```python
from build123d import *

# Parameters (mm, degrees)
F0_W     = 64.9693608284
F0_H     = 45.7421503961
F1_DEPTH = 38.1
F3_DEPTH = 38.1
F4_R     = 6.35
F5_DEPTH = 25.4
F6_R     = 3.175
F7_DEPTH = 25.4


with BuildPart() as f1:
    # F0 (on Front) → F1 (new body)
    with BuildSketch(Plane.XZ):
        with Locations((32.4846804142, 22.8710751981)):
            Rectangle(F0_W, F0_H)
    extrude(amount=-F1_DEPTH)

    # F2 (on face) → F3 (cut)
    with BuildSketch(Plane.XY.offset(45.7421503961)):
        Polygon((38.1, 25.4), (0, 25.4), (0, 0), (64.9693608284, 0), (64.9693608284, 38.1), (38.1, 38.1), align=None)
    extrude(amount=-F3_DEPTH, mode=Mode.SUBTRACT)

    # F4 (on face) → F5 (cut)
    with BuildSketch(Plane.XZ.offset(-25.4)):
        with Locations((12.7, 33.0421503961)):
            Circle(F4_R)
        with BuildLine():
            ThreePointArc((12.6999999513, 45.7421503961), (21.6802561039, 42.0224065344), (25.4, 33.0421503961))
            Line((25.4, 33.0421503961), (25.4, 20.3421503961))
            ThreePointArc((25.4, 20.3421503961), (29.1197438789, 11.361894275), (38.1, 7.6421503961))
            Line((38.1, 7.6421503961), (38.1, 45.7421503961))
            Line((38.1, 45.7421503961), (12.6999999513, 45.7421503961))
        make_face()
        with BuildLine():
            ThreePointArc((0, 33.0421503961), (3.7197438617, 42.0224065), (12.6999999513, 45.7421503961))
            Line((12.6999999513, 45.7421503961), (0, 45.7421503961))
            Line((0, 45.7421503961), (0, 33.0421503961))
        make_face()
    extrude(amount=-F5_DEPTH, mode=Mode.SUBTRACT)

    # F6 (on face) → F7 (cut)
    with BuildSketch(Plane.XY.offset(7.6421503961)):
        with Locations((9.525, 9.525)):
            Circle(F6_R)
        with Locations((55.4443608284, 9.525)):
            Circle(F6_R)
        with Locations((55.4443608284, 28.575)):
            Circle(F6_R)
        with BuildLine():
            ThreePointArc((64.9693608284, 9.525), (62.1795529192, 2.7898079092), (55.4443608284, 0))
            Line((55.4443608284, 0), (64.9693608284, 0))
            Line((64.9693608284, 0), (64.9693608284, 9.525))
        make_face()
        with BuildLine():
            ThreePointArc((9.525, 0), (2.7898079092, 2.7898079092), (0, 9.525))
            Line((0, 9.525), (0, 0))
            Line((0, 0), (9.525, 0))
        make_face()
    extrude(amount=-F7_DEPTH, mode=Mode.SUBTRACT)


solid = f1.part
```
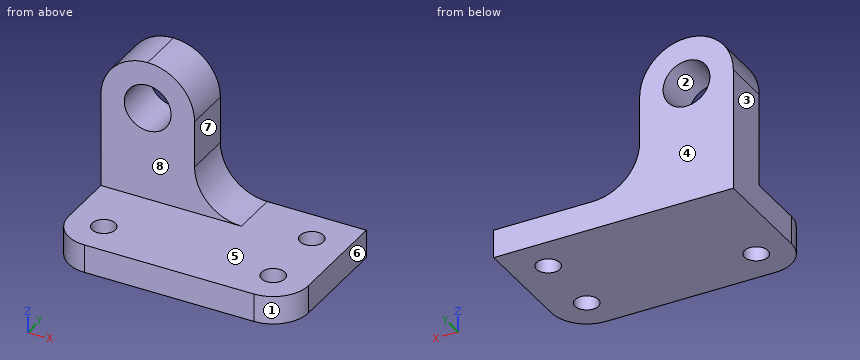
Geometry check sheet. Reference: the model listing, model coordinates, mm. Face numbers are marked on the shaded views. A direction names the side the tool comes from. Round coordinates to 2 decimals unless told otherwise and drop trailing zeros. Loops run counter-clockwise (first coordinate to the right, second up) from the corner with the lowest first, then second, coordinate; pieces in that order, holes last. Notation, with made-up numbers: (26.25, 34) -> (47.25, 34) arc R21 ccw to (47.25, 70) -> close; hole circle Ø9 at (-25.75, -35.75). An arc over 180 degrees is marked (long way). Use a Markdown table: item, result.
(1) Mould release check, pull along X, two halves, no side actions. Record for the marked faces 1, 2, 3 and 4: released by +X, released by -X, zero draft, split by the parting line, or undercut.
Calculated:
| item | result |
|---|---|
| face 1 | released by +X |
| face 2 | undercut |
| face 3 | released by -X |
| face 4 | zero draft |
(2) Sectioned sample at A-A (z = 34). Enter the section's corners in (x, y), then the cut area to 3 significant figures.
Calculated:
| item | result |
|---|---|
| outline | (0.04, 25.4) -> (6.42, 25.4) -> (6.42, 38.1) -> (0.04, 38.1) -> close; (18.98, 25.4) -> (25.36, 25.4) -> (25.36, 38.1) -> (18.98, 38.1) -> close |
| area | 162 mm² |
(3) Sectioned sample at D-D (x = 27.5). Enter the section's corners in (y, z).
Calculated:
| item | result |
|---|---|
| outline | (0, 0) -> (38.1, 0) -> (38.1, 13.35) -> (25.4, 13.35) -> (25.4, 7.64) -> (0, 7.64) -> close |
(4) Go/stop test with flat-tipped pins: P1, Ø8.5, axis at x = 9.525, y = 9.525, coming from the +Z side; P2, Ø6.5, axis at y = 31, z = 25.5, coming from the +X side; P3, Ø19, axis at x = 22, z = 31.5, coming from the -Y side. Record where each tip stops, or that it passes through.
Calculated:
| item | result |
|---|---|
| P1 | z = 7.64 |
| P2 | x = 25.4 |
| P3 | y = 25.4 |
(5) Sectioned sample at C-C (y = 21.5). Enter the section's corners in (x, z), then the cut area to 3 significant figures.
Calculated:
| item | result |
|---|---|
| outline | (0, 0) -> (64.97, 0) -> (64.97, 7.64) -> (0, 7.64) -> close |
| area | 497 mm² |
(6) Sectioned sample at B-B (z = 6.5). Enter the section's corners in (x, y) (3 decimals), then the cut area to 3 significant figures.
Calculated:
| item | result |
|---|---|
| outline | (0, 9.525) arc R9.525 ccw to (9.525, 0) -> (55.444, 0) arc R9.525 ccw to (64.969, 9.525) -> (64.969, 38.1) -> (0, 38.1) -> close; hole circle Ø6.35 at (9.525, 9.525); hole circle Ø6.35 at (55.444, 9.525); hole circle Ø6.35 at (55.444, 28.575) |
| area | 2,340 mm² |
(7) Scan lines: probe 1 along Z at (x, y) = (7.5, 24); probe 2 along X at (y, z) = (31, 21.5); probe 3 along X at (y, z) = (7.5, 6). Record each from-to range of solid material in increasing order.
Calculated:
| item | result |
|---|---|
| probe 1 | 0 to 7.64 |
| probe 2 | 0 to 25.4 |
| probe 3 | 0.22 to 7.08, 11.97 to 53, 57.89 to 64.75 |
(8) Set-up check for the marked faces 5, 6, 7 and 8: record each of +Z, -Z, +X, -X, +Y, -Y from which the full face is reachable in a straight line by a thin tool's end or side.
Calculated:
| item | result |
|---|---|
| face 5 | +Z, +X, -Y |
| face 6 | +Z, -Z, +X, +Y, -Y |
| face 7 | +Z, +X, +Y, -Y |
| face 8 | +Z, +X, -X, -Y |
